Here's how the part is built. I have some questions about the finished solid (model axes, mm). A direction names the side the tool comes from. Give positions to 0.01 mm unless a question says otherwise; leave off trailing zeros. Write each loop counter-clockwise with the first axis right and the second up, starting at its lowest first coordinate (ties: lowest second). Pieces come first, ordered by that corner, then holes. Notation, with made-up numbers: M 85,-30 L 137,-30 A27 ccw 137,-14 Z; hole C 65.5,-31 d2. An arc over 180 degrees is marked long. Answer as CSV lines item,"result". Start each with the question number.
Q1. Suppose I cut it at B-B (x = 11). Write out the boundary of the cut face in (y, z), then the cut area to 3 significant figures.
Q2. Thinking about a two-plate mould opening in Z: for faces 4 (the cylindrical face through (24.386, 0.986, 1.405)), 5 (the cylindrical face through (-10.073, 0.986, 2.387)), 6 (the cylindrical face through (8.928, 0.986, 4.246)), which applies, +Z half, -Z half, draft (parallel to the pull), parting line (faces both ways), or undercut?
Q3. On a 3-axis mill with a long thin cutter (end or side, diameter ignored), from which of +Z, -Z, +X, -X, +Y, -Y can I reach the whole of each face in a straight line? I mean faces 1 (the flat face through (1, 1, 0.566)), 2 (the cylindrical face through (25.94, 0.99, 1.98)), 3 (the flat face through (1, 1, 4.066)). Say none if no direction works.
Q4. For pin 1 (1 mm diameter, centred on x = -2, y = 1.5, fed in from +Z), with a flat end and sliding along its axis, tell me the tip position at first contact or that it passes through.
Q5. If I drill on line 1 along Z through (x, y) = (-3.5, 0.95); line 2 along X through (y, z) = (0.3, -1); line 3 along X through (y, z) = (1.65, -1.5), over which ranges is the centre line in solid material (lowest first)?
Q6. Suppose I cut it at C-C (y = 0.7). Write out the boundary of the cut face in (x, z), then the cut area to 3 significant figures.
Q7. Suppose I cut it at A-A (z = -1.25). Write out the boundary of the cut face in (x, y).
Q8. Suppose I cut it at D-D (x = 4). Write out the boundary of the cut face in (y, z), then the cut area to 3 significant figures.
```python
from build123d import *

# Parameters (mm, degrees)
SKETCH1_R           = 7
SKETCH1_R_2         = 1
BOSS_EXTRUDE1_DEPTH = 2


with BuildPart() as part:
    # Sketch1 → Boss-Extrude1 (new body)
    with BuildSketch(Plane(origin=(0, 0, 0), x_dir=(1, 0, 0), z_dir=(0, 1, 0))):
        with BuildLine():
            Line((-6.410211793, -0.565826241), (8.355574645, -0.565826241))
            ThreePointArc((8.355574645, -0.565826241), (8.921122441, -0.390541761), (9.288406736, 0.07386238))
            ThreePointArc((9.288406736, 0.07386238), (25.945574645, -2.315826241), (9.288406736, -4.705514861))
            ThreePointArc((9.288406736, -4.705514861), (8.921122441, -4.24111072), (8.355574645, -4.065826241))
            Line((8.355574645, -4.065826241), (-6.410211793, -4.065826241))
            ThreePointArc((-6.410211793, -4.065826241), (-10.074425355, -2.315826241), (-6.410211793, -0.565826241))
        make_face()
        with Locations(Location((17.445574645, -2.315826241, 0), (0, 0, 270))):
            Circle(SKETCH1_R, mode=Mode.SUBTRACT)
        with Locations(Location((-7.824425355, -2.315826241, 0), (0, 0, 270))):
            Circle(SKETCH1_R_2, mode=Mode.SUBTRACT)
    extrude(amount=BOSS_EXTRUDE1_DEPTH)


solid = part.part
```
Resolved:
1,outline,"M 0,-3.23 L 2,-3.23 L 2,-0.41 L 0,-0.41 Z; M 0,5.05 L 2,5.05 L 2,7.86 L 0,7.86 Z"
1,area,"11.2 mm^2"
2,face 4,"undercut"
2,face 5,"parting line"
2,face 6,"+Z half"
3,face 1,"-Z, +Y, -Y"
3,face 2,"+Y, -Y"
3,face 3,"+Z, +Y, -Y"
4,pin 1,"z = 4.07"
5,line 1,"0.57 to 4.07"
5,line 2,"9.62 to 11.28, 23.61 to 25.27"
5,line 3,"9.85 to 11.58, 23.31 to 25.04"
6,outline,"M -6.41,0.57 L 8.36,0.57 A1 cw 9.29,-0.07 A8.5 ccw long 9.29,4.71 A1 cw 8.36,4.07 L -6.41,4.07 A2.25 ccw long Z; hole C -7.82,2.32 d2; hole C 17.45,2.32 d14"
6,area,"138 mm^2"
7,outline,"M 9.73,0 L 11.42,0 L 11.42,2 L 9.73,2 Z; M 23.47,0 L 25.16,0 L 25.16,2 L 23.47,2 Z"
8,outline,"M 0,0.57 L 2,0.57 L 2,4.07 L 0,4.07 Z"
8,area,"7.00 mm^2"
